```python
from build123d import *

# Parameters (mm, degrees)
TABAN_FLAN_1_DEPTH         = 50
KES_EKSTR_ZYON1_DEPTH      = 4481.915196698
KES_EKSTR_ZYON1_DEPTH_BACK = 4481.915196698
IZIM2_W                    = 942
IZIM2_H                    = 710
IZIM3_W                    = 11
IZIM3_H                    = 3300
SEKME1_DEPTH               = 50
KES_EKSTR_ZYON2_DEPTH      = 4486.833255929
KES_EKSTR_ZYON2_DEPTH_BACK = 4486.833255929
IZIM4_W                    = 1520
IZIM4_H                    = 310
KES_EKSTR_ZYON3_DEPTH      = 4486.833255929
KES_EKSTR_ZYON3_DEPTH_BACK = 4486.833255929
IZIM6_W                    = 7
IZIM6_H                    = 2435
KES_EKSTR_ZYON4_DEPTH      = 4337.484751501
KES_EKSTR_ZYON4_DEPTH_BACK = 4337.484751501
IZIM7_W                    = 360
IZIM7_H                    = 1550
KES_EKSTR_ZYON5_DEPTH      = 4213.683230436
KES_EKSTR_ZYON5_DEPTH_BACK = 4213.683230436
IZIM8_W                    = 3
IZIM8_H                    = 1550
IZIM8_W_2                  = 58
IZIM8_H_2                  = 885
IZIM9_W                    = 905
IZIM9_H                    = 5
SEKME2_DEPTH               = 50
KES_EKSTR_ZYON6_DEPTH      = 4212.765544282
KES_EKSTR_ZYON6_DEPTH_BACK = 4212.765544282
IZIM10_W                   = 101
IZIM10_H                   = 1555
KES_EKSTR_ZYON7_DEPTH      = 4183.008608313
KES_EKSTR_ZYON7_DEPTH_BACK = 4183.008608313
IZIM11_W                   = 409
IZIM11_H                   = 1555
KES_EKSTR_ZYON8_DEPTH      = 4085.890329005
KES_EKSTR_ZYON8_DEPTH_BACK = 4085.890329005
IZIM13_W                   = 395
IZIM13_H                   = 665


# Sheet-metal steps are written as plain solids
with BuildPart() as part:
    # Çizim1 → Taban-Flanş1 (new body)
    with BuildSketch(Plane.XY):
        Polygon((0, 0), (1427, 0), (1427, 710), (1999, 710), (1999, 4010), (0, 4010), align=None)
    extrude(amount=-TABAN_FLAN_1_DEPTH)

    # Çizim2 → Kes-Ekstrüzyon1 (cut, two sides: drawn at the far end of the back side and taken through both)
    with BuildSketch(Plane.XY.offset(-KES_EKSTR_ZYON1_DEPTH_BACK)):
        with Locations((956, 355)):
            Rectangle(IZIM2_W, IZIM2_H)
    extrude(amount=KES_EKSTR_ZYON1_DEPTH + KES_EKSTR_ZYON1_DEPTH_BACK, mode=Mode.SUBTRACT)

    # Çizim3 → Sekme1 (add)
    with BuildSketch(Plane.XY):
        with Locations((2004.5, 2360)):
            Rectangle(IZIM3_W, IZIM3_H)
    extrude(amount=-SEKME1_DEPTH)

    # Çizim4 → Kes-Ekstrüzyon2 (cut, two sides: drawn at the far end of the back side and taken through both)
    with BuildSketch(Plane.XY.offset(-KES_EKSTR_ZYON2_DEPTH_BACK)):
        with Locations((1250, 865)):
            Rectangle(IZIM4_W, IZIM4_H)
    extrude(amount=KES_EKSTR_ZYON2_DEPTH + KES_EKSTR_ZYON2_DEPTH_BACK, mode=Mode.SUBTRACT)

    # Çizim6 → Kes-Ekstrüzyon3 (cut, two sides: drawn at the far end of the back side and taken through both)
    with BuildSketch(Plane.XY.offset(-KES_EKSTR_ZYON3_DEPTH_BACK)):
        Polygon((440, 2460), (440, 1575), (440, 1020), (490, 1020), (2010, 1020), (2010, 4010), (1650, 4010), (1650, 2460), align=None)
        Polygon((7, 1575), (0, 1575), (0, 0), (485, 0), (485, 710), (490, 710), (490, 1020), (440, 1020), (440, 1575), align=None)
        with Locations((3.5, 2792.5)):
            Rectangle(IZIM6_W, IZIM6_H)
    extrude(amount=KES_EKSTR_ZYON3_DEPTH + KES_EKSTR_ZYON3_DEPTH_BACK, mode=Mode.SUBTRACT)

    # Çizim7 → Kes-Ekstrüzyon4 (cut, two sides: drawn at the far end of the back side and taken through both)
    with BuildSketch(Plane.XY.offset(-KES_EKSTR_ZYON4_DEPTH_BACK)):
        with Locations((1470, 3235)):
            Rectangle(IZIM7_W, IZIM7_H)
    extrude(amount=KES_EKSTR_ZYON4_DEPTH + KES_EKSTR_ZYON4_DEPTH_BACK, mode=Mode.SUBTRACT)

    # Çizim8 → Kes-Ekstrüzyon5 (cut, two sides: drawn at the far end of the back side and taken through both)
    with BuildSketch(Plane.XY.offset(-KES_EKSTR_ZYON5_DEPTH_BACK)):
        Polygon((382, 3385), (7, 3385), (7, 1575), (382, 1575), (382, 2460), align=None)
        with Locations((1288.5, 3235)):
            Rectangle(IZIM8_W, IZIM8_H)
        with Locations((411, 2017.5)):
            Rectangle(IZIM8_W_2, IZIM8_H_2)
    extrude(amount=KES_EKSTR_ZYON5_DEPTH + KES_EKSTR_ZYON5_DEPTH_BACK, mode=Mode.SUBTRACT)

    # Çizim9 → Sekme2 (add)
    with BuildSketch(Plane.XY):
        with Locations((834.5, 2457.5)):
            Rectangle(IZIM9_W, IZIM9_H)
    extrude(amount=-SEKME2_DEPTH)

    # Çizim10 → Kes-Ekstrüzyon6 (cut, two sides: drawn at the far end of the back side and taken through both)
    with BuildSketch(Plane.XY.offset(-KES_EKSTR_ZYON6_DEPTH_BACK)):
        with Locations((1236.5, 3232.5)):
            Rectangle(IZIM10_W, IZIM10_H)
    extrude(amount=KES_EKSTR_ZYON6_DEPTH + KES_EKSTR_ZYON6_DEPTH_BACK, mode=Mode.SUBTRACT)

    # Çizim11 → Kes-Ekstrüzyon7 (cut, two sides: drawn at the far end of the back side and taken through both)
    with BuildSketch(Plane.XY.offset(-KES_EKSTR_ZYON7_DEPTH_BACK)):
        with Locations((981.5, 3232.5)):
            Rectangle(IZIM11_W, IZIM11_H)
    extrude(amount=KES_EKSTR_ZYON7_DEPTH + KES_EKSTR_ZYON7_DEPTH_BACK, mode=Mode.SUBTRACT)

    # Çizim13 → Kes-Ekstrüzyon8 (cut, two sides: drawn at the far end of the back side and taken through both)
    with BuildSketch(Plane.XY.offset(-KES_EKSTR_ZYON8_DEPTH_BACK)):
        with Locations((579.5, 2787.5)):
            Rectangle(IZIM13_W, IZIM13_H)
    extrude(amount=KES_EKSTR_ZYON8_DEPTH + KES_EKSTR_ZYON8_DEPTH_BACK, mode=Mode.SUBTRACT)


solid = part.part
```
Can you work these out from the model? Positions are in its coordinate system, mm. A direction names the side the tool comes from. Coordinates: 2 decimals unless noted, no trailing zeros. Loops run counter-clockwise (first coordinate to the right, second up) from the corner with the lowest first, then second, coordinate; pieces in that order, holes last.
1) For pin 1 (1.5 mm diameter, centred on x = 116, z = -30, fed in from -Y), with a flat end and sliding along its axis, tell me the tip position at first contact or that it passes through.
2) Imagine slicing it at A-A on z = -33. List the corners of the cut face in (x, y) for me.
3) Imagine slicing it at C-C on y = 3207.5. List the corners of the cut face in (x, z) for me, plus the area to 4 significant figures.
4) Which directions (+Z, -Z, +X, -X, +Y, -Y) give clear straight access to the entire face, cutting with the end or side of a thin tool? Please do faces 1 (the flat face through (387, 4010, -25)), 2 (the flat face through (197, 3385, -25)).
5) Imagine slicing it at B-B on x = 300.5. List the corners of the cut face in (y, z) for me, plus the area to 4 significant figures.
6) I need wall thicknesses on probe 1 along X at (y, z) = (3308.5, -4.5); probe 2 along Y at (x, z) = (166, -8). Which ranges of each line are inside material? Lowest first, please.
Completed:
1. pin 1: stops at y = 3385
2. outline: (7, 3385) - (382, 3385) - (382, 3120) - (777, 3120) - (777, 4010) - (7, 4010) - close
3. outline: (382, -50) - (777, -50) - (777, 0) - (382, 0) - close
3. area: 19,750 mm2
4. face 1: +Z, -Z, +X, -X, +Y
4. face 2: +Z, -Z, -X, -Y
5. outline: (3385, -50) - (4010, -50) - (4010, 0) - (3385, 0) - close
5. area: 31,250 mm2
6. probe 1: x = 382 to 777
6. probe 2: y = 3385 to 4010
